Verification items for this drawing (mm, ordinates from the low corner). Round coordinates to 2 decimals unless told otherwise and drop trailing zeros. Write each loop counter-clockwise with the first axis right and the second up, starting at its lowest first coordinate (ties: lowest second). Pieces come first, ordered by that corner, then holes. Notation, with made-up numbers: (-5, -1) -> (47, -1) arc R28 ccw to (47, 26) -> close; hole circle Ø10 at (52.5, 26.5). An arc over 180 degrees is marked (long way). One line per question, with ' | ' between items.
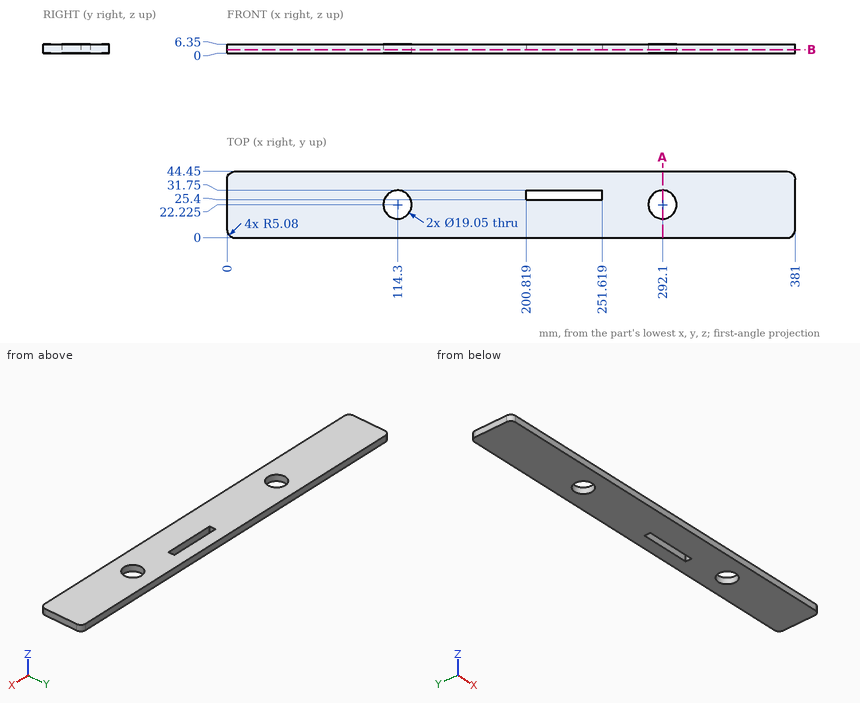
(1) Material ranges on line 1 (X direction, y = 22, z = 1); line 2 (X direction, y = 30, z = 5.5); line 3 (Y direction, x = 114.3, z = 4), recorded low to high.
Resolved:
line 1: x = 0 to 104.78, 123.82 to 282.58, 301.62 to 381 | line 2: x = 0 to 108.8, 119.8 to 200.82, 251.62 to 286.6, 297.6 to 381 | line 3: y = 0 to 12.7, 31.75 to 44.45
(2) Go/stop test with a flat-tipped pin: pin 1 (3 mm diameter, centred on x = 127.5, y = 5.5, fed in from -Z). Record where the tip stops, or that it passes through.
Resolved:
pin 1: stops at z = 0
(3) Sectioned sample at B-B on z = 2.5. Count the separate pieces of the cut face and the enclosed holes in it, then the cut area to 3 significant figures.
Resolved:
separate pieces: 1 | enclosed holes: 3 | area: 16,000 mm2
(4) Sectioned sample at A-A on x = 292.1. Record the cut outline in (y, z).
Resolved:
outline: (0, 0) -> (12.7, 0) -> (12.7, 6.35) -> (0, 6.35) -> close; (31.75, 0) -> (44.45, 0) -> (44.45, 6.35) -> (31.75, 6.35) -> close
